Can you work these out from the model? Positions are in its coordinate system, mm. A direction names the side the tool comes from. Coordinates: 2 decimals unless noted, no trailing zeros. Order: outer loops, then holes, each group sorted by start corner. A loop starts at its lowest first (then second) coordinate and runs counter-clockwise, first axis right, second up. Notation, with made-up numbers: M 40.25,-1 L 58.25,-1 A26 cw 58.25,13 Z; hole C 68,32 d2. An arc over 180 degrees is marked long. Answer as a JSON object with one key per item and string values.
from build123d import *

# Parameters (mm, degrees)
F1_DEPTH = 250


# Not quite as in the source:
# - a feature names something its author has since deleted; it is built from what else it names


with BuildPart() as f1:
    # F0 (on Top) → F1 (new body)
    with BuildSketch(Plane.XY):
        with BuildLine():
            Line((-225.7312981026, 56.6), (-210.7312981026, 56.6))
            ThreePointArc((-210.7312981026, 56.6), (-208.5596069481, 64.1414869616), (-206.1181214741, 71.6))
            Line((-206.1181214741, 71.6), (-225.7312981026, 71.6))
            Line((-225.7312981026, 71.6), (-225.7312981026, 56.6))
        make_face()
        with BuildLine():
            ThreePointArc((206.1181214741, 71.6), (208.5596069481, 64.1414869616), (210.7312981026, 56.6))
            Line((210.7312981026, 56.6), (225.7312981026, 56.6))
            Line((225.7312981026, 56.6), (225.7312981026, 71.6))
            Line((225.7312981026, 71.6), (206.1181214741, 71.6))
        make_face()
        with BuildLine():
            ThreePointArc((-210.7312981026, 56.6), (-28.5453214557, -216.3247665502), (218.2, 0))
            ThreePointArc((218.2, 0), (216.3247665502, 28.5453214557), (210.7312981026, 56.6))
            ThreePointArc((210.7312981026, 56.6), (208.5596069481, 64.1414869616), (206.1181214741, 71.6))
            Line((206.1181214741, 71.6), (190.1675051106, 71.6))
            ThreePointArc((190.1675051106, 71.6), (199.9153283749, 36.3882052424), (203.2, 0))
            ThreePointArc((203.2, 0), (-36.3882052424, -199.9153283749), (-190.1675051106, 71.6))
            Line((-190.1675051106, 71.6), (-206.1181214741, 71.6))
            ThreePointArc((-206.1181214741, 71.6), (-208.5596069481, 64.1414869616), (-210.7312981026, 56.6))
        make_face()
    extrude(amount=F1_DEPTH)


solid = f1.part
Item 1: I'm going to push flat-ended pins straight in: pin 1 (10 mm diameter, centred on x = -158.5, z = 218, fed in from +Y); pin 2 (2 mm diameter, centred on y = -73, z = 56, fed in from -X); pin 3 (2 mm diameter, centred on x = 36, z = 204, fed in from +Y). Where does each tip first touch, or does it pass through?
Answers follow:
{"pin 1": "stops at y = -120.66", "pin 2": "stops at x = -205.98", "pin 3": "stops at y = -199.8"}
Item 2: I want a section at B-B, the plane z = 68. Write out the boundary of the cut face in (x, y), plus the area to 3 significant figures.
Answers follow:
{"outline": "M -225.73,56.6 L -210.73,56.6 A218.2 ccw long 210.73,56.6 L 225.73,56.6 L 225.73,71.6 L 190.17,71.6 A203.2 cw long -190.17,71.6 L -225.73,71.6 Z", "area": "12,600 mm^2"}
Item 3: I want a section at C-C, the plane y = -95.5. Write out the boundary of the cut face in (x, z).
Answers follow:
{"outline": "M -196.19,0 L -179.36,0 L -179.36,250 L -196.19,250 Z; M 179.36,0 L 196.19,0 L 196.19,250 L 179.36,250 Z"}
Item 4: I want a section at D-D, the plane x = 0. Write out the boundary of the cut face in (y, z), plus the area to 3 significant figures.
Answers follow:
{"outline": "M -218.2,0 L -203.2,0 L -203.2,250 L -218.2,250 Z", "area": "3,750 mm^2"}
Item 5: If we mould it in two halves opening along Y, with no side actions, what happens to faces 1 (the flat face through (218, 56.6, 123)), 2 (the flat face through (208, 71.6, 123)), 3 (the flat face through (32, -201, 250))? For each: pulls with the +Y half, pulls with the -Y half, needs draft (parallel to the pull), parting line crosses it, or undercut.
Answers follow:
{"face 1": "undercut", "face 2": "pulls with the +Y half", "face 3": "needs draft"}
Item 6: I want a section at A-A, the plane y = 39. Write out the boundary of the cut face in (x, z).
Answers follow:
{"outline": "M -214.69,0 L -199.42,0 L -199.42,250 L -214.69,250 Z; M 199.42,0 L 214.69,0 L 214.69,250 L 199.42,250 Z"}
Item 7: Please list where these lines run through material, in increasing order: line 1 (X direction, y = 6.5, z = 44); line 2 (X direction, y = -17, z = 72); line 3 (Y direction, x = 0, z = 91.5).
Answers follow:
{"line 1": "x = -218.1 to -203.1, 203.1 to 218.1", "line 2": "x = -217.54 to -202.49, 202.49 to 217.54", "line 3": "y = -218.2 to -203.2"}
Item 8: Which directions (+Z, -Z, +X, -X, +Y, -Y) give clear straight access to the entire face, cutting with the end or side of a thin tool? Please do faces 4 (the flat face through (-218, 56.6, 123)), 5 (the flat face through (225.731, 64, 123)).
Answers follow:
{"face 4": "+Z, -Z, -X", "face 5": "+Z, -Z, +X, +Y, -Y"}
